For this review, take the finished solid that the model builds, in its own axes (mm). A direction names the side the tool comes from. Give positions to 0.01 mm unless a question says otherwise; leave off trailing zeros. Write each loop counter-clockwise with the first axis right and the second up, starting at its lowest first coordinate (ties: lowest second). Pieces come first, ordered by that corner, then holes. Notation, with made-up numbers: M 26.25,75 L 71.25,75 A15 ccw 71.25,98 Z; hole C -36.5,62.25 d6. An arc over 180 degrees is marked long. Use one line per item in the form item = value. Start each with the question number.
Q1. Mouldability with a two-part tool opening along X and no side actions: class faces 1 (the flat face through (2, 35, 10)), 2 (the flat face through (34, 21.5, -2)), 3 (the cylindrical face through (-6, 35, 6)) as released by +X, released by -X, zero draft, split by the parting line, or undercut.
Q2. Tool access review of faces 4 (the flat face through (19.5, 1, 8)), 5 (the flat face through (13, 20.5, -2)), 6 (the flat face through (27, 19, -2)): name each direction out of +Z, -Z, +X, -X, +Y, -Y from which nothing blocks a thin tool from reaching the whole face with its end or side.
Q3. Consider section D-D on x = 31.75. Write out the cut boundary in (y, z), and give its area (3 significant figures).
Q4. Consider section C-C on z = 10. Write out the cut boundary in (x, y).
Q5. Clearance check with flat-ended pins moving along their axes: pin 1 Ø0.9 at (x, y) = (13.5, 1) entering from +Z; pin 2 Ø11.5 at (x, y) = (16, 39) entering from -Z; pin 3 Ø3.5 at (y, z) = (1.5, 3) entering from -X. State where each tip first meets the part, or that it passes through.
Q6. For probe 1 along Y at (x, z) = (7.25, 1.9); probe 2 along X at (y, z) = (23.5, 6); probe 3 along Y at (x, z) = (9, 9), list the stretches that pass through material, from the lowest coordinate up. Write a range as [from, to].
Q7. Consider section A-A on x = 14. Write out the cut boundary in (y, z), and give its area (3 significant figures).
```python
from build123d import *

# Parameters (mm, degrees)
SKETCH1_W                = 39
SKETCH1_H                = 70
BASE_DEPTH               = 4.5
SKETCH2_W                = 4
SKETCH2_H                = 62
WALLS_DEPTH              = 7.5
SKETCH3_W                = 10
SKETCH3_H                = 7.5
PWR_CONNECTOR_HOLE_DEPTH = 4
SKETCH4_W                = 7.5
SKETCH4_H                = 8
GPS_CONNECTOR_HOLE_DEPTH = 4
SKETCH5_R                = 1.25
MOUNTING_HOLES_DEPTH     = 4
GPS_MOUNT_DEPTH          = 4
SKETCH11_W               = 17
SKETCH11_H               = 1
SKETCH11_W_2             = 12
SKETCH11_H_2             = 3
PWR_CABLE_HOLDER1_DEPTH  = 4
SKETCH12_W               = 4
SKETCH12_H               = 2.5
PWR_CABLE_HOLDER2_DEPTH  = 3
PWR_FILLET_R             = 1.5
PWR_FILLET2_R            = 1
PWR_FILLET3_R            = 0.5
GPS_CABLE_HOLDER_DEPTH   = 3
GPS_START                = 1
GPS_FILLET_DEPTH         = 10
GPS_START_2              = 16.5
GPS_FILLET_2_DEPTH       = 4
GPS_START_3              = 9.15727
GPS_FILLET_3_DEPTH       = 8.34273
GPS_FILLET_2_2_R         = 0.5
SKETCH15_R               = 6
BALLON_MOUNT_DEPTH       = 70
SKETCH16_R               = 2.25
BALLOON_MOUNT_HOLE_DEPTH = 70
SKETCH21_R               = 2.25
SAFETY_MOUNT_DEPTH       = 4.5
SKETCH22_W               = 35
SKETCH22_H               = 66
LID_HOLE_DEPTH           = 7.5
SKETCH25_W               = 3.5
SKETCH25_H               = 66
CORRECTION_DEPTH         = 2
SKETCH28_W               = 2
SKETCH28_H               = 2
SMALLER_WALLS_DEPTH      = 2
SKETCH29_W               = 11
SKETCH29_H               = 14
ANTENNA_SPACE_DEPTH      = 1.5


with BuildPart() as part:
    # Sketch1 → Base (new body)
    with BuildSketch(Plane.XY):
        with Locations((19.5, 35)):
            Rectangle(SKETCH1_W, SKETCH1_H)
    extrude(amount=BASE_DEPTH)

    # Sketch2 → Walls (add)
    with BuildSketch(Plane.XY.offset(4.5)):
        Polygon((39, 66), (39, 70), (0, 70), (0, 66), (4, 66), (35, 66), align=None)
        with Locations((37, 35)):
            Rectangle(SKETCH2_W, SKETCH2_H)
        Polygon((4, 66), (0, 66), (0, 0), (4, 0), (4, 4), align=None)
        Polygon((39, 0), (39, 4), (35, 4), (4, 4), (4, 0), align=None)
    extrude(amount=WALLS_DEPTH)

    # Sketch3 → PWR connector hole (cut)
    with BuildSketch(Plane(origin=(0, 4, 0), x_dir=(1, 0, 0), z_dir=(0, 1, 0))):
        with Locations((14.5, -8.25)):
            Rectangle(SKETCH3_W, SKETCH3_H)
    extrude(amount=-PWR_CONNECTOR_HOLE_DEPTH, mode=Mode.SUBTRACT)

    # Sketch4 → GPS connector hole (cut)
    with BuildSketch(Plane.ZY.offset(-35)):
        with Locations((8.25, 18.5)):
            Rectangle(SKETCH4_W, SKETCH4_H)
    extrude(amount=-GPS_CONNECTOR_HOLE_DEPTH, mode=Mode.SUBTRACT)

    # Sketch5 → Mounting holes (cut)
    with BuildSketch(Plane.XY.offset(4.5)):
        with Locations((7.25, 7.25)):
            Circle(SKETCH5_R)
        with Locations(Location((31.75, 7.25, 0), (0, 0, 180))):
            Circle(SKETCH5_R)
        with Locations(Location((7.25, 62.75, 0), (0, 0, 180))):
            Circle(SKETCH5_R)
    extrude(amount=-MOUNTING_HOLES_DEPTH, mode=Mode.SUBTRACT)

    # Sketch7 → GPS mount (add)
    with BuildSketch(Plane(origin=(0, 0, 0), x_dir=(-1, 0, 0), z_dir=(0, 0, -1))):
        Polygon((-39, 1), (-39, 0), (-7, 0), (-7, 18.5), (-39, 18.5), (-39, 17.5), (-8, 17.5), (-8, 1), align=None)
    extrude(amount=GPS_MOUNT_DEPTH)

    # Sketch11 → PWR cable holder1 (add)
    with BuildSketch(Plane(origin=(0, 0, 0), x_dir=(-1, 0, 0), z_dir=(0, 0, -1))):
        Polygon((-5, 0), (-4, 0), (-4, 21.5), (-5, 21.5), (-5, 20.5), align=None)
        with Locations((-13.5, 21)):
            Rectangle(SKETCH11_W, SKETCH11_H)
        with Locations((-33, 20)):
            Rectangle(SKETCH11_W_2, SKETCH11_H_2)
    extrude(amount=PWR_CABLE_HOLDER1_DEPTH)

    # Sketch12 → PWR cable holder2 (cut)
    with BuildSketch(Plane.XZ):
        Polygon((5, 2), (5, 0), (7, 0), (16.5, 0), (16.5, 2), (12.5, 2), align=None)
        with Locations((14.5, 3.25)):
            Rectangle(SKETCH12_W, SKETCH12_H)
    extrude(amount=-PWR_CABLE_HOLDER2_DEPTH, mode=Mode.SUBTRACT)

    # PWR fillet
    pwr_fillet_edges = [part.edges().sort_by_distance(p)[0] for p in [
        (6, 3, 0),
        (14.5, 3, 4.5),
    ]]
    fillet(pwr_fillet_edges, radius=PWR_FILLET_R)

    # PWR fillet2
    pwr_fillet2_edges = [part.edges().sort_by_distance(p)[0] for p in [
        (27, 21.5, -2),
    ]]
    fillet(pwr_fillet2_edges, radius=PWR_FILLET2_R)

    # PWR fillet3
    pwr_fillet3_edges = [part.edges().sort_by_distance(p)[0] for p in [
        (22, 21.5, -2),
        (22, 20.5, -2),
    ]]
    fillet(pwr_fillet3_edges, radius=PWR_FILLET3_R - 0.0001)  # a hair under: the kernel refuses the full size

    # Sketch13 → GPS cable holder (cut)
    with BuildSketch(Plane(origin=(39, 0, 0), x_dir=(0, 0, -1), z_dir=(1, 0, 0))):
        Polygon((-1.156586719, 11), (-2.326586719, 11), (-2.326586719, 1), (0, 1), (0, 11), align=None)
        Polygon((-2.326586719, 11), (-2.326586719, 16.5), (-3.326586719, 16.5), (-3.326586719, 1), (-2.326586719, 1), align=None)
        Polygon((-1.156586719, 20.5), (-2.326586719, 20.5), (-2.326586719, 16.5), (-2.326586719, 11), (-1.156586719, 11), align=None)
        Polygon((-2.326586719, 20.5), (-4.5, 20.5), (-4.5, 16.5), (-3.326586719, 16.5), (-2.326586719, 16.5), align=None)
    extrude(amount=-GPS_CABLE_HOLDER_DEPTH, mode=Mode.SUBTRACT)

    # GPS fillet: read off the stored shape, not the designer's step
    # GPS fillet outline → GPS fillet (cut)
    with BuildSketch(Plane(origin=(0, 0, 0), x_dir=(1, 0, 0), z_dir=(0, 1, 0)).offset(GPS_START)):
        with BuildLine():
            Line((36, -3.326586719), (36, -3.25))
            ThreePointArc((36, -3.25), (35.999412758, -3.288311358), (35.997651584, -3.326586719))
            Line((35.997651584, -3.326586719), (36, -3.326586719))
        make_face()
        with BuildLine():
            Line((36, -1.25), (36, 0))
            Line((36, 0), (34.75, 0))
            ThreePointArc((34.75, 0), (35.633883476, -0.366116524), (36, -1.25))
        make_face()
    extrude(amount=GPS_FILLET_DEPTH, mode=Mode.SUBTRACT)

    # GPS fillet 2 outline → GPS fillet 2 (cut)
    with BuildSketch(Plane(origin=(0, 0, 0), x_dir=(1, 0, 0), z_dir=(0, 1, 0)).offset(GPS_START_2)):
        with BuildLine():
            ThreePointArc((36, -3.25), (35.633883476, -4.133883476), (34.75, -4.5))
            Line((34.75, -4.5), (36, -4.5))
            Line((36, -4.5), (36, -3.25))
        make_face()
        with BuildLine():
            ThreePointArc((35.996504697, -1.156586719), (35.999125868, -1.203260674), (36, -1.25))
            Line((36, -1.25), (36, -1.156586719))
            Line((36, -1.156586719), (35.996504697, -1.156586719))
        make_face()
    extrude(amount=GPS_FILLET_2_DEPTH, mode=Mode.SUBTRACT)

    # GPS fillet 3 outline → GPS fillet 3 (cut)
    with BuildSketch(Plane(origin=(0, 0, 0), x_dir=(1, 0, 0), z_dir=(0, 1, 0)).offset(GPS_START_3)):
        with BuildLine():
            Line((36, -3.326586719), (36, -3.25))
            ThreePointArc((36, -3.25), (35.999412758, -3.288311358), (35.997651584, -3.326586719))
            Line((35.997651584, -3.326586719), (36, -3.326586719))
        make_face()
        with BuildLine():
            ThreePointArc((35.996504697, -1.156586719), (35.999125868, -1.203260674), (36, -1.25))
            Line((36, -1.25), (36, -1.156586719))
            Line((36, -1.156586719), (35.996504697, -1.156586719))
        make_face()
    extrude(amount=GPS_FILLET_3_DEPTH, mode=Mode.SUBTRACT)

    # GPS fillet 2 2
    # the kernel refuses this fillet: 0.5 mm, written as the material it takes off along each edge
    with BuildSketch(Plane(origin=(40.25, 11, 1.156586719), x_dir=(0, 0, -1), z_dir=(-1, 0, 0))) as gps_fillet_2_2_piece_1:
        with BuildLine():
            CenterArc((GPS_FILLET_2_2_R, -GPS_FILLET_2_2_R), GPS_FILLET_2_2_R, 90, 90)
            Line((0, -GPS_FILLET_2_2_R), (0, 0))
            Line((0, 0), (GPS_FILLET_2_2_R, 0))
        make_face()
    extrude(amount=4.25, mode=Mode.SUBTRACT)
    with BuildSketch(Plane(origin=(40.25, 16.5, 3.326586719), x_dir=(0, -1, 0), z_dir=(-1, 0, 0))) as gps_fillet_2_2_piece_2:
        with BuildLine():
            CenterArc((GPS_FILLET_2_2_R, GPS_FILLET_2_2_R), GPS_FILLET_2_2_R, 180, 90)
            Line((0, GPS_FILLET_2_2_R), (0, 0))
            Line((0, 0), (GPS_FILLET_2_2_R, 0))
        make_face()
    extrude(amount=4.25, mode=Mode.SUBTRACT)
    with BuildSketch(Plane(origin=(36, 16.5, 3.326586719), x_dir=(0, -1.0, 5.126796764898245e-10), z_dir=(-1, 0, 0))) as gps_fillet_2_2_piece_3_section:
        with BuildLine():
            CenterArc((GPS_FILLET_2_2_R, GPS_FILLET_2_2_R), GPS_FILLET_2_2_R, 179.999999971, 90)
            Line((GPS_FILLET_2_2_R * 5.12679676753e-10, GPS_FILLET_2_2_R), (0, 0))
            Line((0, 0), (GPS_FILLET_2_2_R, 0))
        make_face()
    gps_fillet_2_2_piece_3 = extrude(amount=1.252348417, mode=Mode.PRIVATE)
    gps_fillet_2_2_piece_3 = gps_fillet_2_2_piece_3 - Plane(origin=(34.749999755, 16.5, 3.249999996), x_dir=(1.0, 0, 2.949740140725451e-09), z_dir=(0, -1, 0)) * Cylinder(1.250000245, 5, mode=Mode.PRIVATE)
    add(gps_fillet_2_2_piece_3, mode=Mode.SUBTRACT)
    with BuildSketch(Plane(origin=(34.746504697, 11, 1.156586719), x_dir=(0, 0, -1), z_dir=(1, 0, 0))) as gps_fillet_2_2_piece_4_section:
        with BuildLine():
            CenterArc((GPS_FILLET_2_2_R, GPS_FILLET_2_2_R), GPS_FILLET_2_2_R, 180, 90)
            Line((-GPS_FILLET_2_2_R * 5.12674791509e-10, GPS_FILLET_2_2_R), (0, 0))
            Line((0, 0), (GPS_FILLET_2_2_R, 0))
        make_face()
    gps_fillet_2_2_piece_4 = extrude(amount=1.253495303, mode=Mode.PRIVATE)
    gps_fillet_2_2_piece_4 = gps_fillet_2_2_piece_4 - Plane(origin=(34.749999998, 11, 1.250000002), x_dir=(1.3197563913171698e-09, 0, -1.0), z_dir=(0, -1, 0)) * Cylinder(1.250000002, 5, mode=Mode.PRIVATE)
    add(gps_fillet_2_2_piece_4, mode=Mode.SUBTRACT)

    # Sketch15 → Ballon mount (add)
    with BuildSketch(Plane.XZ):
        with Locations((0, 6)):
            Circle(SKETCH15_R)
    extrude(amount=-BALLON_MOUNT_DEPTH)

    # Sketch16 → Balloon mount hole (cut)
    with BuildSketch(Plane.XZ):
        with Locations(Location((0, 6, 0), (0, 0, 270))):
            Circle(SKETCH16_R)
    extrude(amount=-BALLOON_MOUNT_HOLE_DEPTH, mode=Mode.SUBTRACT)

    # Sketch21 → Safety mount (cut)
    with BuildSketch(Plane.ZY.offset(6)):
        with Locations((6, 3.5)):
            Circle(SKETCH21_R)
        with Locations((6, 66.5)):
            Circle(SKETCH21_R)
    extrude(amount=-SAFETY_MOUNT_DEPTH, mode=Mode.SUBTRACT)

    # Sketch22 → Lid hole (cut)
    with BuildSketch(Plane.XY.offset(12)):
        with Locations((19.5, 35)):
            Rectangle(SKETCH22_W, SKETCH22_H)
    extrude(amount=-LID_HOLE_DEPTH, mode=Mode.SUBTRACT)

    # Sketch25 → Correction (add)
    with BuildSketch(Plane(origin=(2, 0, 0), x_dir=(0, 0, -1), z_dir=(1, 0, 0))):
        with Locations((-6.25, 35)):
            Rectangle(SKETCH25_W, SKETCH25_H)
    extrude(amount=CORRECTION_DEPTH)

    # Sketch28 → Smaller walls (add)
    with BuildSketch(Plane.XY.offset(4.5)):
        with Locations((38, 21.5)):
            Rectangle(SKETCH28_W, SKETCH28_H)
        with Locations((38, 15.5)):
            Rectangle(SKETCH28_W, SKETCH28_H)
    extrude(amount=SMALLER_WALLS_DEPTH)

    # Sketch29 → Antenna space (cut)
    with BuildSketch(Plane.XY.offset(4.5)):
        with Locations((31.5, 61)):
            Rectangle(SKETCH29_W, SKETCH29_H)
    extrude(amount=-ANTENNA_SPACE_DEPTH, mode=Mode.SUBTRACT)


solid = part.part
```
Working result:
q1.face_1 = undercut
q1.face_2 = zero draft
q1.face_3 = released by -X
q2.face_4 = +Z, -Y
q2.face_5 = -Z
q2.face_6 = -Z, +Y
q3.outline = M 0,-4 L 1,-4 L 1,0 L 17.5,0 L 17.5,-4 L 21.5,-4 L 21.5,0 L 70,0 L 70,12 L 68,12 L 68,3 L 54,3 L 54,4.5 L 8.5,4.5 L 8.5,0.5 L 6,0.5 L 6,4.5 L 2,4.5 L 2,12 L 0,12 Z
q3.area = 334 mm²
q4.outline = M -4.47,0 L 9.5,0 L 9.5,2 L 2,2 L 2,68 L 37,68 L 37,22.5 L 39,22.5 L 39,70 L -4.47,70 Z; M 19.5,0 L 39,0 L 39,14.5 L 37,14.5 L 37,2 L 19.5,2 Z
q5.pin_1 = 0
q5.pin_2 = 0
q5.pin_3 = -5.87
q6.probe_1 = [3, 6], [8.5, 61.5], [64, 70]
q6.probe_2 = [-6, -2.25], [2, 4], [37, 39]
q6.probe_3 = [0, 2], [68, 70]
q7.outline = M 0,-4 L 1,-4 L 1,0 L 0,0 Z; M 3,0 L 17.5,0 L 17.5,-4 L 18.5,-4 L 18.5,0 L 20.5,0 L 20.5,-4 L 21.5,-4 L 21.5,0 L 70,0 L 70,12 L 68,12 L 68,4.5 L 4.5,4.5 A1.5 ccw 3,3 Z
q7.area = 328 mm²
